```python
from build123d import *

# Parameters (mm, degrees)
SKETCH_1_R          = 1.5
EXTRUDE_1_DEPTH     = 1.5
CUT_EXTRUDE_2_DEPTH = 0.8
SKETCH_4_R          = 3
SKETCH_4_R_2        = 1.5
EXTRUDE_2_DEPTH     = 1.6
FILLET_1_R          = 1
CHAMFER_1_SIZE      = 2


with BuildPart() as part:
    # Эскиз1 → Бобышка-Вытянуть1 (new body)
    with BuildSketch(Plane.XY):
        with BuildLine():
            Line((-3, 14.696938457), (-3, 8.696938457))
            Line((-3, 8.696938457), (3, 8.696938457))
            Line((3, 8.696938457), (3, 14.696938457))
            Line((3, 14.696938457), (19.657078674, 16.594796577))
            ThreePointArc((19.657078674, 16.594796577), (21.287556094, 16.919662188), (22.841677521, 17.51017118))
            ThreePointArc((22.841677521, 17.51017118), (29.425159504, 15.327651899), (27.493638863, 8.666206601))
            Line((27.493638863, 8.666206601), (14.696938457, 3))
            Line((14.696938457, 3), (8.696938457, 3))
            Line((8.696938457, 3), (8.696938457, -3))
            Line((8.696938457, -3), (14.696938457, -3))
            ThreePointArc((14.696938457, -3), (13.858192988, -5.740251485), (12.513625189, -8.270984502))
            Line((12.513625189, -8.270984502), (8.270984502, -4.028343815))
            Line((8.270984502, -4.028343815), (4.028343815, -8.270984502))
            Line((4.028343815, -8.270984502), (8.270984502, -12.513625189))
            ThreePointArc((8.270984502, -12.513625189), (5.740251485, -13.858192988), (3, -14.696938457))
            Line((3, -14.696938457), (3, -8.696938457))
            Line((3, -8.696938457), (-3, -8.696938457))
            Line((-3, -8.696938457), (-3, -14.696938457))
            ThreePointArc((-3, -14.696938457), (-5.740251485, -13.858192988), (-8.270984502, -12.513625189))
            Line((-8.270984502, -12.513625189), (-4.028343815, -8.270984502))
            Line((-4.028343815, -8.270984502), (-8.270984502, -4.028343815))
            Line((-8.270984502, -4.028343815), (-12.513625189, -8.270984502))
            ThreePointArc((-12.513625189, -8.270984502), (-13.858192988, -5.740251485), (-14.696938457, -3))
            Line((-14.696938457, -3), (-8.696938457, -3))
            Line((-8.696938457, -3), (-8.696938457, 3))
            Line((-8.696938457, 3), (-14.696938457, 3))
            Line((-14.696938457, 3), (-27.014954435, 8.423980045))
            ThreePointArc((-27.014954435, 8.423980045), (-29.543661072, 15.086898192), (-22.841677521, 17.51017118))
            ThreePointArc((-22.841677521, 17.51017118), (-21.287556094, 16.919662188), (-19.657078674, 16.594796577))
            Line((-19.657078674, 16.594796577), (-3, 14.696938457))
        make_face()
        with Locations((-25, 13)):
            Circle(SKETCH_1_R, mode=Mode.SUBTRACT)
        with Locations((25, 13)):
            Circle(SKETCH_1_R, mode=Mode.SUBTRACT)
        Polygon((4.028343815, 8.270984502), (8.270984502, 4.028343815), (12.513625189, 8.270984502), (8.270984502, 12.513625189), align=None, mode=Mode.SUBTRACT)
        Polygon((-8.270984502, 4.028343815), (-4.028343815, 8.270984502), (-8.270984502, 12.513625189), (-12.513625189, 8.270984502), align=None, mode=Mode.SUBTRACT)
    extrude(amount=EXTRUDE_1_DEPTH)

    # Эскиз3 → Вырез-Вытянуть2 (cut)
    with BuildSketch(Plane(origin=(0, 0, 0), x_dir=(-1, 0, 0), z_dir=(0, 0, -1))):
        Polygon((-4, 7.696938457), (-4, 9.656854249), (-7.87527044, 13.53212469), (-13.53212469, 7.87527044), (-9.656854249, 4), (-7.696938457, 4), (-7.696938457, 3.188176298), (-3.188176298, 7.696938457), align=None)
        Polygon((-8.270984502, 4.028343815), (-12.513625189, 8.270984502), (-8.270984502, 12.513625189), (-4.028343815, 8.270984502), align=None, mode=Mode.SUBTRACT)
        Polygon((-2.614130252, 8.270984502), (-4, 9.656854249), (-4, 7.696938457), (-3.188176298, 7.696938457), align=None)
        Polygon((-3, 14.696938457), (-4, 14.81087549), (-4, 9.656854249), (-2.614130252, 8.270984502), (-3.188176298, 7.696938457), (3.188176298, 7.696938457), (2.614130252, 8.270984502), (4, 9.656854249), (4, 14.81087549), (3, 14.696938457), (3, 8.696938457), (-3, 8.696938457), align=None)
        Polygon((4, 7.696938457), (4, 9.656854249), (2.614130252, 8.270984502), (3.188176298, 7.696938457), align=None)
        Polygon((7.87527044, 13.53212469), (4, 9.656854249), (4, 7.696938457), (3.188176298, 7.696938457), (7.696938457, 3.188176298), (7.696938457, 4), (9.656854249, 4), (13.53212469, 7.87527044), align=None)
        Polygon((4.028343815, 8.270984502), (8.270984502, 12.513625189), (12.513625189, 8.270984502), (8.270984502, 4.028343815), align=None, mode=Mode.SUBTRACT)
        Polygon((7.696938457, 4), (7.696938457, 3.188176298), (8.270984502, 2.614130252), (9.656854249, 4), align=None)
        with BuildLine():
            Line((8.270984502, 2.614130252), (7.696938457, 3.188176298))
            Line((7.696938457, 3.188176298), (7.696938457, -3.188176298))
            Line((7.696938457, -3.188176298), (8.270984502, -2.614130252))
            Line((8.270984502, -2.614130252), (9.656854249, -4))
            Line((9.656854249, -4), (14.456832295, -4))
            ThreePointArc((14.456832295, -4), (14.585458075, -3.502058358), (14.696938457, -3))
            Line((14.696938457, -3), (8.696938457, -3))
            Line((8.696938457, -3), (8.696938457, 3))
            Line((8.696938457, 3), (14.696938457, 3))
            Line((14.696938457, 3), (15.137314264, 3.193910253))
            Line((15.137314264, 3.193910253), (15.137314264, 4))
            Line((15.137314264, 4), (9.656854249, 4))
            Line((9.656854249, 4), (8.270984502, 2.614130252))
        make_face()
        Polygon((8.270984502, -2.614130252), (7.696938457, -3.188176298), (7.696938457, -4), (9.656854249, -4), align=None)
        with BuildLine():
            Line((7.696938457, -4), (7.696938457, -3.188176298))
            Line((7.696938457, -3.188176298), (3.188176298, -7.696938457))
            Line((3.188176298, -7.696938457), (4, -7.696938457))
            Line((4, -7.696938457), (4, -9.656854249))
            Line((4, -9.656854249), (7.394097025, -13.050951275))
            ThreePointArc((7.394097025, -13.050951275), (7.837147099, -12.789805525), (8.270984502, -12.513625189))
            Line((8.270984502, -12.513625189), (4.028343815, -8.270984502))
            Line((4.028343815, -8.270984502), (8.270984502, -4.028343815))
            Line((8.270984502, -4.028343815), (12.513625189, -8.270984502))
            ThreePointArc((12.513625189, -8.270984502), (12.789805525, -7.837147099), (13.050951275, -7.394097025))
            Line((13.050951275, -7.394097025), (9.656854249, -4))
            Line((9.656854249, -4), (7.696938457, -4))
        make_face()
        with BuildLine():
            Line((3.188176298, -7.696938457), (-3.188176298, -7.696938457))
            Line((-3.188176298, -7.696938457), (-2.614130252, -8.270984502))
            Line((-2.614130252, -8.270984502), (-4, -9.656854249))
            Line((-4, -9.656854249), (-4, -14.456832295))
            ThreePointArc((-4, -14.456832295), (-3.502058358, -14.585458075), (-3, -14.696938457))
            Line((-3, -14.696938457), (-3, -8.696938457))
            Line((-3, -8.696938457), (3, -8.696938457))
            Line((3, -8.696938457), (3, -14.696938457))
            ThreePointArc((3, -14.696938457), (3.502058358, -14.585458075), (4, -14.456832295))
            Line((4, -14.456832295), (4, -9.656854249))
            Line((4, -9.656854249), (2.614130252, -8.270984502))
            Line((2.614130252, -8.270984502), (3.188176298, -7.696938457))
        make_face()
        Polygon((4, -7.696938457), (3.188176298, -7.696938457), (2.614130252, -8.270984502), (4, -9.656854249), align=None)
        Polygon((-2.614130252, -8.270984502), (-3.188176298, -7.696938457), (-4, -7.696938457), (-4, -9.656854249), align=None)
        with BuildLine():
            Line((-3.188176298, -7.696938457), (-7.696938457, -3.188176298))
            Line((-7.696938457, -3.188176298), (-7.696938457, -4))
            Line((-7.696938457, -4), (-9.656854249, -4))
            Line((-9.656854249, -4), (-13.050951275, -7.394097025))
            ThreePointArc((-13.050951275, -7.394097025), (-12.789805525, -7.837147099), (-12.513625189, -8.270984502))
            Line((-12.513625189, -8.270984502), (-8.270984502, -4.028343815))
            Line((-8.270984502, -4.028343815), (-4.028343815, -8.270984502))
            Line((-4.028343815, -8.270984502), (-8.270984502, -12.513625189))
            ThreePointArc((-8.270984502, -12.513625189), (-7.837147099, -12.789805525), (-7.394097025, -13.050951275))
            Line((-7.394097025, -13.050951275), (-4, -9.656854249))
            Line((-4, -9.656854249), (-4, -7.696938457))
            Line((-4, -7.696938457), (-3.188176298, -7.696938457))
        make_face()
        Polygon((-7.696938457, -4), (-7.696938457, -3.188176298), (-8.270984502, -2.614130252), (-9.656854249, -4), align=None)
        with BuildLine():
            Line((-7.696938457, -3.188176298), (-7.696938457, 3.188176298))
            Line((-7.696938457, 3.188176298), (-8.270984502, 2.614130252))
            Line((-8.270984502, 2.614130252), (-9.656854249, 4))
            Line((-9.656854249, 4), (-15.137314264, 4))
            Line((-15.137314264, 4), (-15.137314264, 3.194992477))
            Line((-15.137314264, 3.194992477), (-14.696938457, 3))
            Line((-14.696938457, 3), (-8.696938457, 3))
            Line((-8.696938457, 3), (-8.696938457, -3))
            Line((-8.696938457, -3), (-14.696938457, -3))
            ThreePointArc((-14.696938457, -3), (-14.585458075, -3.502058358), (-14.456832295, -4))
            Line((-14.456832295, -4), (-9.656854249, -4))
            Line((-9.656854249, -4), (-8.270984502, -2.614130252))
            Line((-8.270984502, -2.614130252), (-7.696938457, -3.188176298))
        make_face()
        Polygon((-8.270984502, 2.614130252), (-7.696938457, 3.188176298), (-7.696938457, 4), (-9.656854249, 4), align=None)
    extrude(amount=-CUT_EXTRUDE_2_DEPTH, mode=Mode.SUBTRACT)

    # Эскиз4 → Бобышка-Вытянуть2 (add)
    with BuildSketch(Plane(origin=(0, 0, 0), x_dir=(-1, 0, 0), z_dir=(0, 0, -1))):
        with Locations((25, 13)):
            Circle(SKETCH_4_R)
        with Locations((25, 13)):
            Circle(SKETCH_4_R_2, mode=Mode.SUBTRACT)
        with Locations((-25, 13)):
            Circle(SKETCH_4_R)
        with Locations((-25, 13)):
            Circle(SKETCH_4_R_2, mode=Mode.SUBTRACT)
    extrude(amount=EXTRUDE_2_DEPTH)

    # Скругление1
    fillet_1_edges = [part.edges().sort_by_distance(p)[0] for p in [
        (-22, 13, 0),
        (28, 13, 0),
    ]]
    fillet(fillet_1_edges, radius=FILLET_1_R)

    # Фаска1
    chamfer_1_edges = [part.edges().sort_by_distance(p)[0] for p in [
        (-26.5, 13, 1.5),
        (23.5, 13, 1.5),
    ]]
    chamfer(chamfer_1_edges, length=CHAMFER_1_SIZE)


solid = part.part
```
Geometry check sheet. Reference: the model listing, model coordinates, mm. A direction names the side the tool comes from. Round coordinates to 2 decimals unless told otherwise and drop trailing zeros. Loops run counter-clockwise (first coordinate to the right, second up) from the corner with the lowest first, then second, coordinate; pieces in that order, holes last. Notation, with made-up numbers: (81.5, 12) - (100.5, 12) arc R21 cw to (100.5, 45) - close; hole circle Ø5 at (-2.5, 75). An arc over 180 degrees is marked (long way). Write item = value, one per line. Start each with the question number.
1. Section check B-B on x = -1. Enter the section's corners in (y, z), then the cut area to 3 significant figures.
2. Thickness scan on line 1 (X direction, y = 13, z = -0.95); line 2 (Y direction, x = -25, z = -0.9); line 3 (X direction, y = -7.5, z = 0.85). Record the ranges inside material, lowest first.
3. Section check D-D on x = 6. Enter the section's corners in (y, z), then the cut area to 3 significant figures.
4. Mould release check, pull along X, two halves, no side actions. Record for faces 1 (the face through (5.78, -13.84, 0.91)), 2 (the face through (-20.77, 5.674, 0.74)), 3 (the face through (-11.45, 15.66, 0.74)): released by +X, released by -X, zero draft, split by the parting line, or undercut.
5. Set-up check for faces 4 (the face through (-13.84, -5.78, 0.91)), 5 (the face through (-10.42, 6.18, 1.15)), 6 (the face through (-5.965, 11.622, 0.394)): record each of +Z, -Z, +X, -X, +Y, -Y from which the full face is reachable in a straight line by a thin tool's end or side.
6. Section check A-A on y = -5.5. Enter the section's corners in (x, z).
7. Depth check by flat-ended pin: pin 1 (0.9 mm diameter, centred on y = 1, z = 0.5, fed in from -X); pin 2 (0.8 mm diameter, centred on y = 12, z = 1.5, fed in from +X); pin 3 (0.8 mm diameter, centred on y = -12, z = 1, fed in from -X). Enter the tip coordinate at first touch or a pass-through.
8. Section check C-C on x = -11. Enter the section's corners in (y, z).
Working result:
q1.outline = (-8.7, 0.8) - (-7.7, 0.8) - (-7.7, 0) - (7.7, 0) - (7.7, 0.8) - (8.7, 0.8) - (8.7, 1.5) - (-8.7, 1.5) - close
q1.area = 24.5 mm^2
q2.line_1 = -28 to -26.5, -23.5 to -22, 22 to 23.5, 26.5 to 28
q2.line_2 = 9.99 to 11.5, 14.5 to 16.01
q2.line_3 = -12.99 to -11.74, -4.8 to 4.8, 11.74 to 12.99
q3.outline = (-13.75, 0) - (-11.66, 0) - (-11.66, 0.8) - (-10.24, 0.8) - (-10.24, 1.5) - (-13.75, 1.5) - close; (-6.3, 0.8) - (-4.89, 0.8) - (-4.89, 0) - (4.89, 0) - (4.89, 0.8) - (6.3, 0.8) - (6.3, 1.5) - (-6.3, 1.5) - close; (10.24, 0.8) - (11.66, 0.8) - (11.66, 0) - (15.04, 0) - (15.04, 1.5) - (10.24, 1.5) - close
q3.area = 26.8 mm^2
q4.face_1 = released by +X
q4.face_2 = released by -X
q4.face_3 = undercut
q5.face_4 = +Z, -Z, -X, -Y
q5.face_5 = +Z, -Z
q5.face_6 = -Z
q6.outline = (-13.96, 0) - (-11.16, 0) - (-11.16, 0.8) - (-9.74, 0.8) - (-9.74, 1.5) - (-13.96, 1.5) - close; (-6.8, 0.8) - (-5.39, 0.8) - (-5.39, 0) - (5.39, 0) - (5.39, 0.8) - (6.8, 0.8) - (6.8, 1.5) - (-6.8, 1.5) - close; (9.74, 0.8) - (11.16, 0.8) - (11.16, 0) - (13.96, 0) - (13.96, 1.5) - (9.74, 1.5) - close
q7.pin_1 = -8.7
q7.pin_2 = 29.96
q7.pin_3 = -8.16
q8.outline = (-6.76, 0.8) - (-5.34, 0.8) - (-5.34, 0) - (-4, 0) - (-4, 0.8) - (-3, 0.8) - (-3, 1.5) - (-6.76, 1.5) - close; (3, 0.8) - (4, 0.8) - (4, 0) - (5.34, 0) - (5.34, 0.8) - (6.76, 0.8) - (6.76, 1.5) - (3, 1.5) - close; (9.78, 0.8) - (10.41, 0.8) - (10.41, 0) - (15.61, 0) - (15.61, 1.5) - (9.78, 1.5) - close
